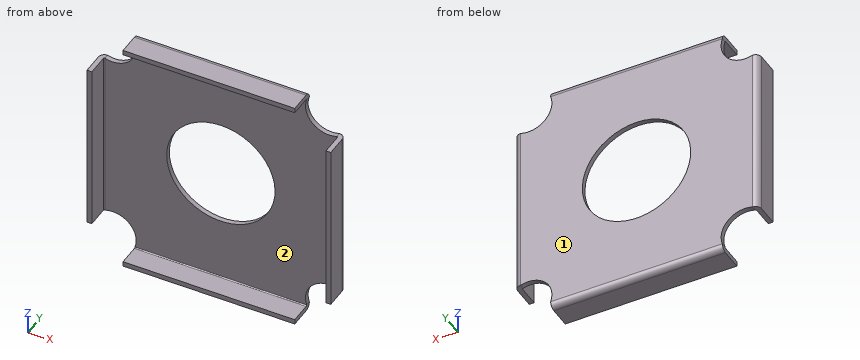
```python
from build123d import *

# Parameters (mm, degrees)
SKETCH3_R                 = 38.1
BASE_FLANGE1_DEPTH        = 3.4163
EDGE_FLANGE1_DEPTH        = 120.765617952
EDGE_FLANGE1_BEND_DEPTH   = 120.765617952
EDGE_FLANGE1_BEND_2_DEPTH = 120.765617952
EDGE_FLANGE1_BEND_3_DEPTH = 120.765617952


# Sheet-metal steps are written as plain solids
with BuildPart() as part:
    # Sketch3 → Base-Flange1 (new body)
    with BuildSketch(Plane(origin=(0, 0, 0), x_dir=(1, 0, 0), z_dir=(0, 1, 0))):
        with BuildLine():
            Line((-60.382808976, 81.5594), (60.382808976, 81.5594))
            ThreePointArc((60.382808976, 81.5594), (64.390963201, 64.390963201), (81.5594, 60.382808976))
            Line((81.5594, 60.382808976), (81.5594, -60.382808976))
            ThreePointArc((81.5594, -60.382808976), (64.390963201, -64.390963201), (60.382808976, -81.5594))
            Line((60.382808976, -81.5594), (-60.382808976, -81.5594))
            ThreePointArc((-60.382808976, -81.5594), (-64.390963201, -64.390963201), (-81.5594, -60.382808976))
            Line((-81.5594, -60.382808976), (-81.5594, 60.382808976))
            ThreePointArc((-81.5594, 60.382808976), (-64.390963201, 64.390963201), (-60.382808976, 81.5594))
        make_face()
        with Locations(Location((0, 0, 0), (0, 0, 270))):
            Circle(SKETCH3_R, mode=Mode.SUBTRACT)
    extrude(amount=-BASE_FLANGE1_DEPTH)

    # Edge-Flange1 section (across the edge) → Edge-Flange1 (add)
    with BuildSketch(Plane(origin=(60.382808976, -3.4163, 82.296), x_dir=(0, 0, -1), z_dir=(-1, 0, 0))):
        with BuildLine():
            Line((-3.4163, 0.7366), (-3.4163, 15.6337))
            Line((-3.4163, 15.6337), (0, 15.6337))
            Line((0, 15.6337), (0, 0.7366))
            ThreePointArc((0, 0.7366), (0.215745145, 0.215745145), (0.7366, 0))
            Line((0.7366, 0), (0.7366, -3.4163))
            ThreePointArc((0.7366, -3.4163), (-2.199943752, -2.199943752), (-3.4163, 0.7366))
        make_face()
    extrude(amount=EDGE_FLANGE1_DEPTH)

    # Edge-Flange1 section 2 (across the edge) → Edge-Flange1 bend (add)
    with BuildSketch(Plane(origin=(82.296, -3.4163, -60.382808976), x_dir=(-1, 0, 0), z_dir=(0, 0, 1))):
        with BuildLine():
            Line((-3.4163, 0.7366), (-3.4163, 15.6337))
            Line((-3.4163, 15.6337), (0, 15.6337))
            Line((0, 15.6337), (0, 0.7366))
            ThreePointArc((0, 0.7366), (0.215745145, 0.215745145), (0.7366, 0))
            Line((0.7366, 0), (0.7366, -3.4163))
            ThreePointArc((0.7366, -3.4163), (-2.199943752, -2.199943752), (-3.4163, 0.7366))
        make_face()
    extrude(amount=EDGE_FLANGE1_BEND_DEPTH)

    # Edge-Flange1 section 3 (across the edge) → Edge-Flange1 bend 2 (add)
    with BuildSketch(Plane(origin=(-60.382808976, -3.4163, -82.296), x_dir=(0, 0, 1), z_dir=(1, 0, 0))):
        with BuildLine():
            Line((-3.4163, 0.7366), (-3.4163, 15.6337))
            Line((-3.4163, 15.6337), (0, 15.6337))
            Line((0, 15.6337), (0, 0.7366))
            ThreePointArc((0, 0.7366), (0.215745145, 0.215745145), (0.7366, 0))
            Line((0.7366, 0), (0.7366, -3.4163))
            ThreePointArc((0.7366, -3.4163), (-2.199943752, -2.199943752), (-3.4163, 0.7366))
        make_face()
    extrude(amount=EDGE_FLANGE1_BEND_2_DEPTH)

    # Edge-Flange1 section 4 (across the edge) → Edge-Flange1 bend 3 (add)
    with BuildSketch(Plane(origin=(-82.296, -3.4163, 60.382808976), x_dir=(1, 0, 0), z_dir=(0, 0, -1))):
        with BuildLine():
            Line((-3.4163, 0.7366), (-3.4163, 15.6337))
            Line((-3.4163, 15.6337), (0, 15.6337))
            Line((0, 15.6337), (0, 0.7366))
            ThreePointArc((0, 0.7366), (0.215745145, 0.215745145), (0.7366, 0))
            Line((0.7366, 0), (0.7366, -3.4163))
            ThreePointArc((0.7366, -3.4163), (-2.199943752, -2.199943752), (-3.4163, 0.7366))
        make_face()
    extrude(amount=EDGE_FLANGE1_BEND_3_DEPTH)


solid = part.part
```
Source: CAD feature listing. Evaluate the final solid. Frame: model axes, mm. Face numbers are marked on the shaded views. Give positions to 0.01 mm unless a question says otherwise; leave off trailing zeros. Write each loop counter-clockwise with the first axis right and the second up, starting at its lowest first coordinate (ties: lowest second). Pieces come first, ordered by that corner, then holes.
1. Pull-direction query (X, two-part tool) for the marked faces 1 and 2; classes: +X half, -X half, draft (parallel to the pull), parting line (faces both ways), or undercut.
2. Section query D-D (z = 48.5). Return the cut outline in (x, y).
3. Section query A-A (y = -8.5). Return the cut outline in (x, z).
4. Section query B-B (z = 0). Return the cut outline in (x, y).
5. Section query C-C (x = 0). Return the cut outline in (y, z).
6. First-contact query: pin 1 (3.5 mm diameter, centred on y = -5.5, z = 84.5, fed in from +X); pin 2 (10 mm diameter, centred on x = 31.5, z = 28, fed in from -Y); pin 3 (3.5 mm diameter, centred on y = -6.5, z = -83.5, fed in from -X); pin 4 (8 mm diameter, centred on y = -3, z = 16.5, fed in from +X). Flat tips, straight axial feed; report the tip coordinate or a pass-through.
7. Material intervals for line 1 along X through (y, z) = (-4.25, 32); line 2 along Y through (x, z) = (63, 52.5), sorted ascending.
Output values:
1. face 1: draft
1. face 2: undercut
2. outline: (-85.71, -19.05) - (-82.3, -19.05) - (-82.3, -4.15) arc R0.74 cw to (-81.56, -3.42) - (81.56, -3.42) arc R0.74 cw to (82.3, -4.15) - (82.3, -19.05) - (85.71, -19.05) - (85.71, -4.15) arc R4.15 ccw to (81.56, 0) - (-81.56, 0) arc R4.15 ccw to (-85.71, -4.15) - close
3. outline: (-85.71, -60.38) - (-82.3, -60.38) - (-82.3, 60.38) - (-85.71, 60.38) - close; (-60.38, -85.71) - (60.38, -85.71) - (60.38, -82.3) - (-60.38, -82.3) - close; (-60.38, 82.3) - (60.38, 82.3) - (60.38, 85.71) - (-60.38, 85.71) - close; (82.3, -60.38) - (85.71, -60.38) - (85.71, 60.38) - (82.3, 60.38) - close
4. outline: (-85.71, -19.05) - (-82.3, -19.05) - (-82.3, -4.15) arc R0.74 cw to (-81.56, -3.42) - (-38.1, -3.42) - (-38.1, 0) - (-81.56, 0) arc R4.15 ccw to (-85.71, -4.15) - close; (38.1, -3.42) - (81.56, -3.42) arc R0.74 cw to (82.3, -4.15) - (82.3, -19.05) - (85.71, -19.05) - (85.71, -4.15) arc R4.15 ccw to (81.56, 0) - (38.1, 0) - close
5. outline: (-19.05, -85.71) - (-4.15, -85.71) arc R4.15 ccw to (0, -81.56) - (0, -38.1) - (-3.42, -38.1) - (-3.42, -81.56) arc R0.74 cw to (-4.15, -82.3) - (-19.05, -82.3) - close; (-19.05, 82.3) - (-4.15, 82.3) arc R0.74 cw to (-3.42, 81.56) - (-3.42, 38.1) - (0, 38.1) - (0, 81.56) arc R4.15 ccw to (-4.15, 85.71) - (-19.05, 85.71) - close
6. pin 1: stops at x = 60.38
6. pin 2: stops at y = -3.42
6. pin 3: stops at x = -60.38
6. pin 4: stops at x = 85.71
7. line 1: x = -85.71 to -82.3, 82.3 to 85.71
7. line 2: y = -3.42 to 0
